```python
from build123d import *

# Parameters (mm, degrees)
SKETCH1_R           = 23
BOSS_EXTRUDE1_DEPTH = 120
SKETCH2_R           = 14.5
CUT_EXTRUDE1_DEPTH  = 120
CUT_EXTRUDE2_DEPTH  = 2.5
SKETCH5_R           = 2.25
CUT_EXTRUDE3_DEPTH  = 10
BOSS_EXTRUDE2_START = -7
SKETCH6_R           = 14.5
BOSS_EXTRUDE2_DEPTH = 7
SKETCH7_R           = 4
CUT_EXTRUDE4_DEPTH  = 15
CUT_EXTRUDE6_DEPTH  = 25
CUT_EXTRUDE7_DEPTH  = 25


with BuildPart() as part:
    # Sketch1 → Boss-Extrude1 (new body)
    with BuildSketch(Plane(origin=(0, 0, 0), x_dir=(1, 0, 0), z_dir=(0, 1, 0))):
        with Locations(Location((0, 0, 0), (0, 0, 270))):
            Circle(SKETCH1_R)
    extrude(amount=BOSS_EXTRUDE1_DEPTH)

    # Sketch2 → Cut-Extrude1 (cut)
    with BuildSketch(Plane(origin=(0, 120, 0), x_dir=(1, 0, 0), z_dir=(0, 1, 0))):
        with Locations(Location((0, 0, 0), (0, 0, 270))):
            Circle(SKETCH2_R)
    extrude(amount=-CUT_EXTRUDE1_DEPTH, mode=Mode.SUBTRACT)

    # Sketch4 → Cut-Extrude2 (cut)
    with BuildSketch(Plane(origin=(0, 120, 0), x_dir=(1, 0, 0), z_dir=(0, 1, 0))):
        Polygon((-17.5, 4), (-20.964101615, 2), (-20.964101615, -2), (-17.5, -4), (-14.035898385, -2), (-14.035898385, 2), align=None)
        Polygon((14.035898385, 2), (17.5, 4), (20.964101615, 2), (20.964101615, -2), (17.5, -4), (14.035898385, -2), align=None)
    extrude(amount=-CUT_EXTRUDE2_DEPTH, mode=Mode.SUBTRACT)

    # Sketch5 → Cut-Extrude3 (cut)
    with BuildSketch(Plane(origin=(0, 117.5, 0), x_dir=(1, 0, 0), z_dir=(0, 1, 0))):
        with Locations(Location((-17.5, 0, 0), (0, 0, 270))):
            Circle(SKETCH5_R)
        with Locations(Location((17.5, 0, 0), (0, 0, 90))):
            Circle(SKETCH5_R)
    extrude(amount=-CUT_EXTRUDE3_DEPTH, mode=Mode.SUBTRACT)

    # Sketch6 → Boss-Extrude2 (add)
    with BuildSketch(Plane(origin=(0, 0, 0), x_dir=(-1, 0, 0), z_dir=(0, -1, 0)).offset(BOSS_EXTRUDE2_START)):
        with Locations(Location((0, 0, 0), (0, 0, 188.620433548))):
            Circle(SKETCH6_R)
    extrude(amount=BOSS_EXTRUDE2_DEPTH)

    # Sketch7 → Cut-Extrude4 (cut)
    with BuildSketch(Plane.XZ):
        with Locations(Location((0, 0, 0), (0, 0, 270))):
            Circle(SKETCH7_R)
    extrude(amount=-CUT_EXTRUDE4_DEPTH, mode=Mode.SUBTRACT)

    # Sketch8 → Cut-Extrude6 (cut)
    with BuildSketch(Plane(origin=(0, 120, 0), x_dir=(1, 0, 0), z_dir=(0, 1, 0))):
        with BuildLine():
            Line((-10, 10.5), (-10, 17.5))
            Line((-10, 17.5), (10, 17.5))
            Line((10, 17.5), (10, 10.5))
            ThreePointArc((10, 10.5), (0, 14.5), (-10, 10.5))
        make_face()
    extrude(amount=-CUT_EXTRUDE6_DEPTH, mode=Mode.SUBTRACT)

    # Sketch9 → Cut-Extrude7 (cut)
    with BuildSketch(Plane(origin=(0, 120, 0), x_dir=(1, 0, 0), z_dir=(0, 1, 0))):
        Polygon((0, 17.5), (-5, 17.5), (-5, 20.5), (5, 20.5), (5, 17.5), align=None)
    extrude(amount=-CUT_EXTRUDE7_DEPTH, mode=Mode.SUBTRACT)


solid = part.part
```
Work out the finished part from the listing and answer in its coordinate system (mm). Coordinates: 2 decimals unless noted, no trailing zeros. Loops run counter-clockwise (first coordinate to the right, second up) from the corner with the lowest first, then second, coordinate; pieces in that order, holes last. Notation, with made-up numbers: (71.25, 36) - (119.25, 36) arc R17 cw to (119.25, 52) - close; hole circle Ø7 at (32.5, 61). An arc over 180 degrees is marked (long way). Use a Markdown table: item, result.
Item 1: Find section C-C, the plane y = 74. Determine the outline of the cut face in (x, z), and give its area (3 significant figures).
Evaluation:
| item | result |
|---|---|
| outline | circle Ø46 at (0, 0); hole circle Ø29 at (0, 0) |
| area | 1,000 mm2 |
Item 2: Find section D-D, the plane z = 13. Determine the outline of the cut face in (x, y).
Evaluation:
| item | result |
|---|---|
| outline | (-18.97, 0) - (18.97, 0) - (18.97, 120) - (6.42, 120) - (6.42, 7) - (-6.42, 7) - (-6.42, 120) - (-18.97, 120) - close |
Item 3: Given pin 1 Ø1.3 at (x, z) = (18, 0.5) entering from +Y; pin 2 Ø3 at (y, z) = (40.5, 12.5) entering from +X; pin 3 Ø17.5 at (x, z) = (0, 0) entering from +Y; pin 4 Ø7 at (x, z) = (0, 0) entering from -Y, each flat-ended and moving along its own axis, determine where each tip first touches the part or whether it passes through.
Evaluation:
| item | result |
|---|---|
| pin 1 | stops at y = 107.5 |
| pin 2 | stops at x = 20.2 |
| pin 3 | stops at y = 7 |
| pin 4 | passes through |
Item 4: Find section B-B, the plane x = 0. Determine the outline of the cut face in (y, z), and give its area (3 significant figures).
Evaluation:
| item | result |
|---|---|
| outline | (0, -23) - (120, -23) - (120, -20.5) - (95, -20.5) - (95, -14.5) - (7, -14.5) - (7, -4) - (0, -4) - close; (0, 4) - (7, 4) - (7, 14.5) - (120, 14.5) - (120, 23) - (0, 23) - close |
| area | 2,040 mm2 |
Item 5: Find section A-A, the plane z = 0. Determine the outline of the cut face in (x, y), and give its area (3 significant figures).
Evaluation:
| item | result |
|---|---|
| outline | (-23, 0) - (-4, 0) - (-4, 7) - (-14.5, 7) - (-14.5, 117.5) - (-15.25, 117.5) - (-15.25, 107.5) - (-19.75, 107.5) - (-19.75, 117.5) - (-20.96, 117.5) - (-20.96, 120) - (-23, 120) - close; (4, 0) - (23, 0) - (23, 120) - (20.96, 120) - (20.96, 117.5) - (19.75, 117.5) - (19.75, 107.5) - (15.25, 107.5) - (15.25, 117.5) - (14.5, 117.5) - (14.5, 7) - (4, 7) - close |
| area | 2,060 mm2 |
Item 6: Consider probe 1 along X at (y, z) = (109, 0); probe 2 along X at (y, z) = (114.5, -18); probe 3 along Y at (x, z) = (-3.5, -7.5). Determine where each line is inside the solid, lowest interval first. Write a range as from..to.
Evaluation:
| item | result |
|---|---|
| probe 1 | x = -23..-19.75, -15.25..-14.5, 14.5..15.25, 19.75..23 |
| probe 2 | x = -14.32..-5, 5..14.32 |
| probe 3 | y = 0..7 |
